Design review of the part built by this model. Coordinates are the model's own, in mm. Face numbers are marked on the shaded views. A direction names the side the tool comes from. Coordinates: 2 decimals unless noted, no trailing zeros. Loops run counter-clockwise (first coordinate to the right, second up) from the corner with the lowest first, then second, coordinate; pieces in that order, holes last. Notation, with made-up numbers: (63.5, 18.25) -> (82.5, 18.25) arc R24 ccw to (82.5, 34.25) -> close; hole circle Ø8 at (60, -0.5). An arc over 180 degrees is marked (long way). Use CSV: the item, a comma, the result in double quotes.
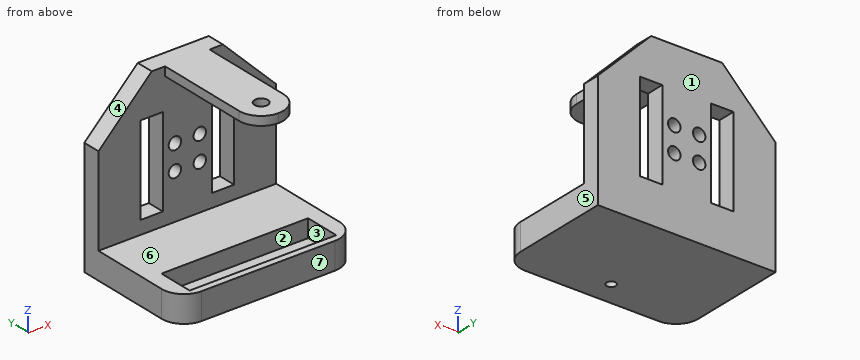
```python
from build123d import *

# Parameters (mm, degrees)
SCHIZZO3_W                   = 40
SCHIZZO3_H                   = 27
ESTRUSIONE_ESTRUSIONE1_DEPTH = 6
SCHIZZO4_W                   = 33
SCHIZZO4_H                   = 8
TAGLIO_ESTRUSIONE1_DEPTH     = 4
SCHIZZO5_R                   = 1.05
TAGLIO_ESTRUSIONE2_DEPTH     = 25.459149617
SCHIZZO6_W                   = 40
SCHIZZO6_H                   = 4
ESTRUSIONE_ESTRUSIONE2_DEPTH = 32
SCHIZZO7_W                   = 10
SCHIZZO7_H                   = 2
ESTRUSIONE_ESTRUSIONE3_DEPTH = 26
SCHIZZO8_R                   = 1.4
SCHIZZO8_W                   = 5
SCHIZZO8_H                   = 20
TAGLIO_ESTRUSIONE3_DEPTH     = 53.383203415
RACCORDO1_R                  = 5
TAGLIO_ESTRUSIONE4_REACH     = 46.365
SCHIZZO9_R                   = 1.5


with BuildPart() as part:
    # Schizzo3 → Estrusione-Estrusione1 (new body)
    with BuildSketch(Plane.XY):
        Rectangle(SCHIZZO3_W, SCHIZZO3_H)
    extrude(amount=ESTRUSIONE_ESTRUSIONE1_DEPTH)

    # Schizzo4 → Taglio-Estrusione1 (cut)
    with BuildSketch(Plane.XY.offset(6)):
        with Locations((0, -8)):
            Rectangle(SCHIZZO4_W, SCHIZZO4_H)
    extrude(amount=-TAGLIO_ESTRUSIONE1_DEPTH, mode=Mode.SUBTRACT)

    # Schizzo5 → Taglio-Estrusione2 (cut, through all)
    with BuildSketch(Plane.XY.offset(2)):
        with Locations((0, -8)):
            Circle(SCHIZZO5_R)
    extrude(amount=-TAGLIO_ESTRUSIONE2_DEPTH, mode=Mode.SUBTRACT)

    # Schizzo6 → Estrusione-Estrusione2 (add)
    with BuildSketch(Plane.XY.offset(6)):
        with Locations((0, 11.5)):
            Rectangle(SCHIZZO6_W, SCHIZZO6_H)
    extrude(amount=ESTRUSIONE_ESTRUSIONE2_DEPTH)

    # Schizzo7 → Estrusione-Estrusione3 (add)
    with BuildSketch(Plane.XZ.offset(-9.5)):
        with Locations((0, 37)):
            Rectangle(SCHIZZO7_W, SCHIZZO7_H)
    extrude(amount=ESTRUSIONE_ESTRUSIONE3_DEPTH)

    # Schizzo8 → Taglio-Estrusione3 (cut, through all)
    with BuildSketch(Plane(origin=(0, 13.5, 0), x_dir=(1, 0, 0), z_dir=(0, 1, 0))):
        with Locations(Location((-2.8, -16.2, 0), (0, 0, 270))):
            Circle(SCHIZZO8_R)
        with Locations(Location((-2.8, -21.8, 0), (0, 0, 270))):
            Circle(SCHIZZO8_R)
        with Locations(Location((2.8, -21.8, 0), (0, 0, 270))):
            Circle(SCHIZZO8_R)
        with Locations(Location((2.8, -16.2, 0), (0, 0, 270))):
            Circle(SCHIZZO8_R)
        with Locations((8, -19)):
            Rectangle(SCHIZZO8_W, SCHIZZO8_H)
        with Locations((-8, -19)):
            Rectangle(SCHIZZO8_W, SCHIZZO8_H)
        Polygon((-20, -26), (-8, -38), (-20, -38), align=None)
        Polygon((8, -38), (20, -38), (20, -26), align=None)
    extrude(amount=-TAGLIO_ESTRUSIONE3_DEPTH, mode=Mode.SUBTRACT)

    # Raccordo1
    raccordo1_edges = [part.edges().sort_by_distance(p)[0] for p in [
        (-5, -16.5, 37),
        (5, -16.5, 37),
        (20, -13.5, 3),
        (-20, -13.5, 3),
    ]]
    fillet(raccordo1_edges, radius=RACCORDO1_R - 0.0001)  # a hair under: the kernel refuses the full size

    # Schizzo9 → Taglio-Estrusione4 (cut, up to next)
    with BuildSketch(Plane(origin=(0, 0, 36), x_dir=(-1, 0, 0), z_dir=(0, 0, -1)), mode=Mode.PRIVATE) as taglio_estrusione4_sk1:
        with Locations((0, -11.5)):
            Circle(SCHIZZO9_R)
    taglio_estrusione4_tool1 = extrude(taglio_estrusione4_sk1.sketch, amount=-TAGLIO_ESTRUSIONE4_REACH, mode=Mode.PRIVATE) & part.part
    add(taglio_estrusione4_tool1.solids().sort_by_distance((0, -11.5, 36))[0], mode=Mode.SUBTRACT)


solid = part.part
```
Item 1: Add section B-B (z = 27). Give the boundary of the cut face in (x, y).
Checked values:
outline,"(-19, 9.5) -> (-10.5, 9.5) -> (-10.5, 13.5) -> (-19, 13.5) -> close; (-5.5, 9.5) -> (5.5, 9.5) -> (5.5, 13.5) -> (-5.5, 13.5) -> close; (10.5, 9.5) -> (19, 9.5) -> (19, 13.5) -> (10.5, 13.5) -> close"
Item 2: Draft analysis for pull direction X (two halves, no side actions). For the marked faces 1, 2, 3 and 4, state which applies: pulls with the +X half, pulls with the -X half, needs draft (parallel to the pull), parting line crosses it, or undercut.
Checked values:
face 1,"needs draft"
face 2,"undercut"
face 3,"undercut"
face 4,"pulls with the -X half"
Item 3: Machinability: for the marked faces 5, 6 and 7, which of the approach directions +Z, -Z, +X, -X, +Y, -Y give a long, thin tool a straight path to every point of the face, cutting with its end or side? Answer none if there is none.
Checked values:
face 5,"+Z, -Z, +X, +Y, -Y"
face 6,"+X, -X, -Y"
face 7,"-Z, +X, -X, -Y"
Item 4: Add section A-A (z = 16.2). Give the boundary of the cut face in (x, y), then the cut area to 3 significant figures.
Checked values:
outline,"(-20, 9.5) -> (-10.5, 9.5) -> (-10.5, 13.5) -> (-20, 13.5) -> close; (-5.5, 9.5) -> (-4.2, 9.5) -> (-4.2, 13.5) -> (-5.5, 13.5) -> close; (-1.4, 9.5) -> (1.4, 9.5) -> (1.4, 13.5) -> (-1.4, 13.5) -> close; (4.2, 9.5) -> (5.5, 9.5) -> (5.5, 13.5) -> (4.2, 13.5) -> close; (10.5, 9.5) -> (20, 9.5) -> (20, 13.5) -> (10.5, 13.5) -> close"
area,"97.6 mm^2"
Item 5: Clearance check with flat-ended pins moving along their axes: pin 1 (2 mm diameter, centred on x = 8.5, y = 12, fed in from +Z); pin 2 (6 mm diameter, centred on y = 4, z = 29, fed in from -X); pin 3 (4 mm diameter, centred on x = -6.5, z = 26, fed in from -Y); pin 4 (5 mm diameter, centred on x = 4.5, z = 3, fed in from -Y). State where each tip first meets the part, or that it passes through.
Checked values:
pin 1,"z = 38"
pin 2,"through"
pin 3,"y = 9.5"
pin 4,"y = -13.5"
Item 6: To check wall thickness, follow line 1 along X through (y, z) = (10.9, 16.2); line 2 along Z through (x, y) = (-4.5, 6.25); line 3 along Y through (x, z) = (0, 1.05). State the ranges of each line that lie inside material, in increasing order.
Checked values:
line 1,"-20 to -10.5, -5.5 to -4.2, -1.4 to 1.4, 4.2 to 5.5, 10.5 to 20"
line 2,"0 to 6, 36 to 38"
line 3,"-13.5 to -9.05, -6.95 to 13.5"
Item 7: Add section D-D (x = 7). Give the boundary of the cut face in (y, z), then the cut area to 3 significant figures.
Checked values:
outline,"(-13.5, 0) -> (13.5, 0) -> (13.5, 9) -> (9.5, 9) -> (9.5, 6) -> (-4, 6) -> (-4, 2) -> (-12, 2) -> (-12, 6) -> (-13.5, 6) -> close; (9.5, 29) -> (13.5, 29) -> (13.5, 38) -> (9.5, 38) -> close"
area,"178 mm^2"
Item 8: Add section C-C (y = 7). Give the boundary of the cut face in (x, z).
Checked values:
outline,"(-20, 0) -> (20, 0) -> (20, 6) -> (-20, 6) -> close; (-5, 36) -> (5, 36) -> (5, 38) -> (-5, 38) -> close"
